The listing builds one solid part. Answer for the finished solid, in the listing's coordinates (mm). Coordinates: 2 decimals unless noted, no trailing zeros. Loops run counter-clockwise (first coordinate to the right, second up) from the corner with the lowest first, then second, coordinate; pieces in that order, holes last. Notation, with made-up numbers: (53.25, -33.75) - (104.25, -33.75) arc R23 cw to (104.25, -1.75) - close; hole circle Ø1 at (69, -18.75). An arc over 180 degrees is marked (long way). Return JSON: item names as keys, results as strings. Group by question number.
1. Section D-D (x = -62) is taken. Write down the section's boundary in (y, z), and give its area (3 significant figures).
2. Section C-C (y = 0.55) is taken. State how many separate pieces and enclosed holes the cut face has, and give its area (3 significant figures).
3. Find the intervals of material crossed by line 1 along X through (y, z) = (1.8, -157); line 2 along Z through (x, y) = (-117, 1.5); line 3 along X through (y, z) = (2.8, -123.5), in increasing order.
4. Section A-A (x = -74.1) is taken. Write down the section's boundary in (y, z).
5. The mould has two halves that part along Z. Classify faces 1 (the face through (-75.3, 1.5, -121.5)), 2 (the face through (-61, 3, -81)), 3 (the face through (-75.3, 1.5, -111.5)): pulls with the +Z half, pulls with the -Z half, needs draft (parallel to the pull), parting line crosses it, or undercut.
6. Section B-B (z = -109.9) is taken. Write down the section's boundary in (x, y).
```python
from build123d import *

# Parameters (mm, degrees)
SKETCH1_W           = 120
SKETCH1_H           = 160
SKETCH1_R           = 1.5
SKETCH1_R_2         = 2
SKETCH1_W_2         = 41.2
SKETCH1_H_2         = 20.2
BOSS_EXTRUDE1_DEPTH = 3


with BuildPart() as part:
    # Sketch1 → Boss-Extrude1 (new body)
    with BuildSketch(Plane(origin=(0, 0, 0), x_dir=(1, 0, 0), z_dir=(0, 1, 0))):
        with Locations((-60, 80)):
            Rectangle(SKETCH1_W, SKETCH1_H)
        with Locations(Location((-117, 157, 0), (0, 0, 270))):
            Circle(SKETCH1_R, mode=Mode.SUBTRACT)
        with Locations(Location((-3, 157, 0), (0, 0, 270))):
            Circle(SKETCH1_R, mode=Mode.SUBTRACT)
        with Locations(Location((-117, 3, 0), (0, 0, 270))):
            Circle(SKETCH1_R, mode=Mode.SUBTRACT)
        with Locations(Location((-3, 3, 0), (0, 0, 270))):
            Circle(SKETCH1_R, mode=Mode.SUBTRACT)
        with Locations(Location((-74.1, 119.9, 0), (0, 0, 270))):
            Circle(SKETCH1_R_2, mode=Mode.SUBTRACT)
        with Locations(Location((-74.1, 109.9, 0), (0, 0, 270))):
            Circle(SKETCH1_R_2, mode=Mode.SUBTRACT)
        with Locations(Location((-24.9, 119.9, 0), (0, 0, 270))):
            Circle(SKETCH1_R_2, mode=Mode.SUBTRACT)
        with Locations(Location((-24.9, 109.9, 0), (0, 0, 270))):
            Circle(SKETCH1_R_2, mode=Mode.SUBTRACT)
        with Locations((-49.5, 114.9)):
            Rectangle(SKETCH1_W_2, SKETCH1_H_2, mode=Mode.SUBTRACT)
    extrude(amount=BOSS_EXTRUDE1_DEPTH)


solid = part.part
```
The answers:
{
 "1": {"outline": "(0, -160) - (3, -160) - (3, -125) - (0, -125) - close; (0, -104.8) - (3, -104.8) - (3, 0) - (0, 0) - close", "area": "419 mm2"},
 "2": {"separate pieces": "1", "enclosed holes": "9", "area": "18,300 mm2"},
 "3": {"line 1": "x = -120 to -118.5, -115.5 to -4.5, -1.5 to 0", "line 2": "z = -160 to -158.5, -155.5 to -4.5, -1.5 to 0", "line 3": "x = -120 to -70.1, -28.9 to 0"},
 "4": {"outline": "(0, -160) - (3, -160) - (3, -121.9) - (0, -121.9) - close; (0, -117.9) - (3, -117.9) - (3, -111.9) - (0, -111.9) - close; (0, -107.9) - (3, -107.9) - (3, 0) - (0, 0) - close"},
 "5": {"face 1": "undercut", "face 2": "needs draft", "face 3": "undercut"},
 "6": {"outline": "(-120, 0) - (-76.1, 0) - (-76.1, 3) - (-120, 3) - close; (-72.1, 0) - (-70.1, 0) - (-70.1, 3) - (-72.1, 3) - close; (-28.9, 0) - (-26.9, 0) - (-26.9, 3) - (-28.9, 3) - close; (-22.9, 0) - (0, 0) - (0, 3) - (-22.9, 3) - close"}
}
